```python
from build123d import *

# Parameters (mm, degrees)
SKETCH1_R           = 11.1125
BOSS_EXTRUDE1_DEPTH = 5.55625
SKETCH2_R           = 7.000000001
CUT_EXTRUDE1_DEPTH  = 5.55625
FILLET1_R           = 10
SKETCH3_R           = 2.250000001
CUT_EXTRUDE2_DEPTH  = 6.35
SKETCH4_R           = 2.5
CUT_EXTRUDE3_DEPTH  = 40


with BuildPart() as part:
    # Sketch1 → Boss-Extrude1 (new body)
    with BuildSketch(Plane.XY):
        with BuildLine():
            Line((-65, 43), (85, 43))
            Line((85, 43), (85, -43))
            Line((85, -43), (-65, -43))
            ThreePointArc((-65, -43), (-108, 0), (-65, 43))
        make_face()
        with Locations((-65, 0)):
            Circle(SKETCH1_R, mode=Mode.SUBTRACT)
    extrude(amount=BOSS_EXTRUDE1_DEPTH)

    # Sketch2 → Cut-Extrude1 (cut)
    with BuildSketch(Plane.XY.offset(5.55625)):
        with Locations((33.66639768, 0)):
            Circle(SKETCH2_R)
    extrude(amount=-CUT_EXTRUDE1_DEPTH, mode=Mode.SUBTRACT)

    # Fillet1
    fillet1_edges = [part.edges().sort_by_distance(p)[0] for p in [
        (85, 43, 2.778125),
        (85, -43, 2.778125),
    ]]
    fillet(fillet1_edges, radius=FILLET1_R)

    # Sketch3 → Cut-Extrude2 (cut)
    with BuildSketch(Plane.XY.offset(5.55625)):
        with Locations((78.66639768, 30)):
            Circle(SKETCH3_R)
        with Locations((78.66639768, -30)):
            Circle(SKETCH3_R)
        with Locations((-11.33360232, 30)):
            Circle(SKETCH3_R)
        with Locations((-11.33360232, -30)):
            Circle(SKETCH3_R)
    extrude(amount=-CUT_EXTRUDE2_DEPTH, mode=Mode.SUBTRACT)

    # Sketch4 → Cut-Extrude3 (cut)
    with BuildSketch(Plane.XY.offset(5.55625)):
        with Locations((0, 17.5)):
            Circle(SKETCH4_R)
        with Locations((0, -17.5)):
            Circle(SKETCH4_R)
    extrude(amount=-CUT_EXTRUDE3_DEPTH, mode=Mode.SUBTRACT)


solid = part.part
```
Geometry: final body of the model. Coordinates: model frame, mm. Coordinates: 2 decimals unless noted, no trailing zeros. Order: outer loops, then holes, each group sorted by start corner. A loop starts at its lowest first (then second) coordinate and runs counter-clockwise, first axis right, second up. Notation, with made-up numbers: M 79.5,78 L 108.5,78 A25 ccw 108.5,108 Z; hole C 6,-35 d2. An arc over 180 degrees is marked long. Answer in a Markdown table with one row per item. Add a question column.
Q1. Section query C-C on z = 1.7. Count the separate pieces of the cut face and the enclosed holes in it, and give its area (3 significant figures).
Q2. Section query A-A on y = 0. Return the cut outline in (x, z).
Q3. Mould query, pull axis X, two halves, no side actions, for faces 1 (the cylindrical face through (-107.99, -0.95, 2.74)), 2 (the cylindrical face through (28.11, -4.26, 2.82)), 3 (the flat face through (-10, 1, 5.556)), 4 (the cylindrical face through (81.99, 40.15, 2.82)). Classes: released by +X, released by -X, zero draft, split by the parting line, or undercut.
Q4. Line query: L1, parallel to Y at x = 0, z = 1.15; L2, parallel to Y at x = 2, z = 0.55; L3, parallel to Y at x = -68.5, z = 1.2. Output: solid intervals per line, ascending.
Q5. Section query D-D on y = 17.5. Return the cut outline in (x, z).
Q6. Section query B-B on x = 0. Return the cut outline in (y, z), and give its area (3 significant figures).
Q7. Contact query for flat-ended pins moving along their axis: P1, Ø6, axis at x = 78.67, y = -30, coming from the +Z side; P2, Ø12.5, axis at x = 33.67, y = 0, coming from the +Z side; P3, Ø1, axis at y = -13, z = 2, coming from the -X side; P4, Ø2, axis at x = -86.5, z = 2, coming from the +Y side. Output: stop coordinate, or through.
Completed:
| question | item | result |
|---|---|---|
| 1 | separate pieces | 1 |
| 1 | enclosed holes | 8 |
| 1 | area | 15,100 mm2 |
| 2 | outline | M -108,0 L -76.11,0 L -76.11,5.56 L -108,5.56 Z; M -53.89,0 L 26.67,0 L 26.67,5.56 L -53.89,5.56 Z; M 40.67,0 L 85,0 L 85,5.56 L 40.67,5.56 Z |
| 3 | face 1 | released by -X |
| 3 | face 2 | undercut |
| 3 | face 3 | zero draft |
| 3 | face 4 | released by +X |
| 4 | L1 | y = -43 to -20, -15 to 15, 20 to 43 |
| 4 | L2 | y = -43 to -19, -16 to 16, 19 to 43 |
| 4 | L3 | y = -42.86 to -10.55, 10.55 to 42.86 |
| 5 | outline | M -104.28,0 L -2.5,0 L -2.5,5.56 L -104.28,5.56 Z; M 2.5,0 L 85,0 L 85,5.56 L 2.5,5.56 Z |
| 6 | outline | M -43,0 L -20,0 L -20,5.56 L -43,5.56 Z; M -15,0 L 15,0 L 15,5.56 L -15,5.56 Z; M 20,0 L 43,0 L 43,5.56 L 20,5.56 Z |
| 6 | area | 422 mm2 |
| 7 | P1 | stops at z = 5.56 |
| 7 | P2 | passes through |
| 7 | P3 | stops at x = -106.14 |
| 7 | P4 | stops at y = 37.8 |
